Check sheet for the drawn part. Datum: minimum x, y, z corner. Units: mm. A direction names the side the tool comes from. Coordinates: 2 decimals unless noted, no trailing zeros. Order: outer loops, then holes, each group sorted by start corner. A loop starts at its lowest first (then second) coordinate and runs counter-clockwise, first axis right, second up. Notation, with made-up numbers: (87, 27.25) -> (96, 27.25) arc R15 cw to (96, 38.25) -> close; hole circle Ø3 at (-31, -21). An arc over 180 degrees is marked (long way). Answer as CSV lines item,"result".
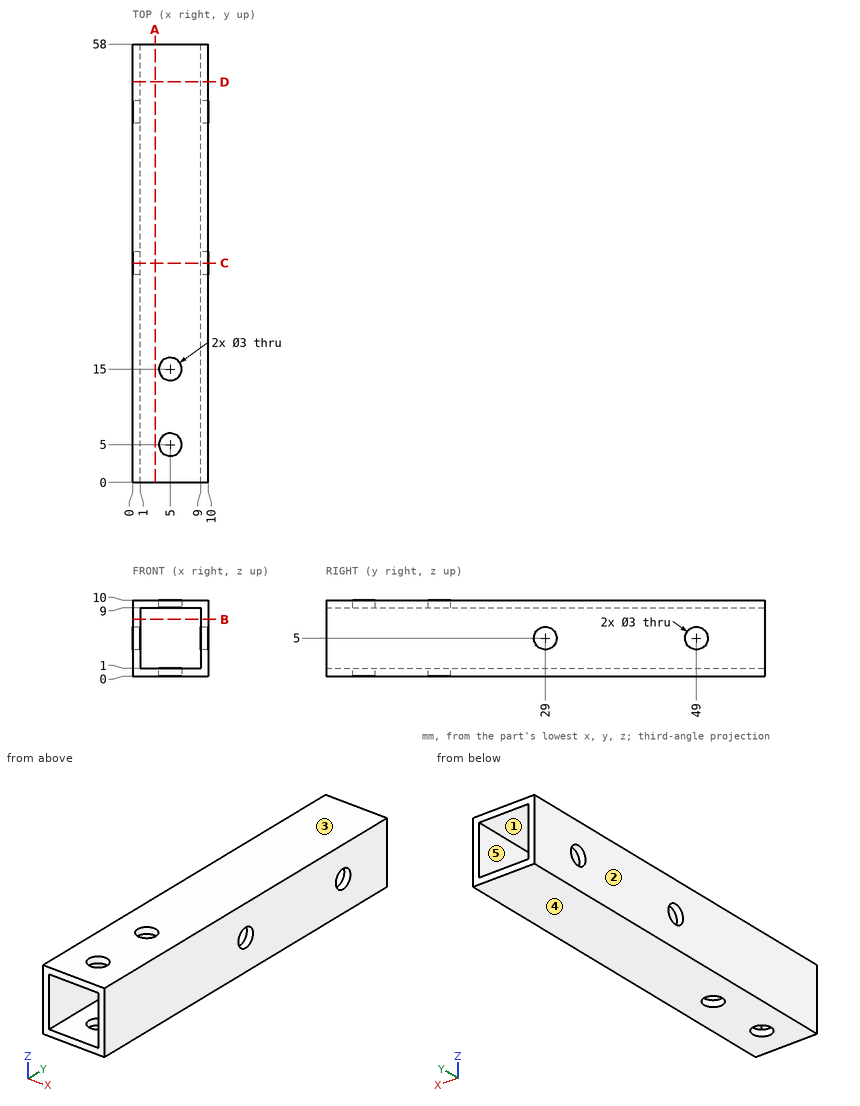
Item 1: Section check B-B, the plane z = 7.5. Record the boundary of the cut face in (x, y), plus the area to 3 significant figures.
Answer list:
outline,"(0, 0) -> (1, 0) -> (1, 58) -> (0, 58) -> close; (9, 0) -> (10, 0) -> (10, 58) -> (9, 58) -> close"
area,"116 mm2"
Item 2: Release check for a two-part mould opening along Z. For the marked faces 3, 4 and 5 record: +Z half, -Z half, draft (parallel to the pull), parting line (faces both ways), or undercut.
Answer list:
face 3,"+Z half"
face 4,"-Z half"
face 5,"undercut"
Item 3: Thickness scan on line 1 (Y direction, x = 9.7, z = 5); line 2 (Z direction, x = 4, y = 46.5). Record the ranges inside material, lowest first.
Answer list:
line 1,"0 to 27.5, 30.5 to 47.5, 50.5 to 58"
line 2,"0 to 1, 9 to 10"
Item 4: Section check D-D, the plane y = 53. Record the boundary of the cut face in (x, z), plus the area to 3 significant figures.
Answer list:
outline,"(0, 0) -> (10, 0) -> (10, 10) -> (0, 10) -> close; hole (1, 1) -> (9, 1) -> (9, 9) -> (1, 9) -> close"
area,"36.0 mm2"
Item 5: Section check A-A, the plane x = 3. Record the boundary of the cut face in (y, z).
Answer list:
outline,"(0, 0) -> (58, 0) -> (58, 1) -> (0, 1) -> close; (0, 9) -> (58, 9) -> (58, 10) -> (0, 10) -> close"
Item 6: Tool access check on the marked faces 1 and 2. Record the directions out of +Z, -Z, +X, -X, +Y, -Y that give a thin tool (end or side, any length) a straight path to the whole face; none if there is none.
Answer list:
face 1,"+Y, -Y"
face 2,"+Z, -Z, -X, +Y, -Y"
Item 7: Section check C-C, the plane y = 29. Record the boundary of the cut face in (x, z), plus the area to 3 significant figures.
Answer list:
outline,"(0, 0) -> (10, 0) -> (10, 3.5) -> (9, 3.5) -> (9, 1) -> (1, 1) -> (1, 3.5) -> (0, 3.5) -> close; (0, 6.5) -> (1, 6.5) -> (1, 9) -> (9, 9) -> (9, 6.5) -> (10, 6.5) -> (10, 10) -> (0, 10) -> close"
area,"30.0 mm2"
Item 8: Depth check by flat-ended pin: pin 1 Ø6 at (x, z) = (2, 9) entering from -Y; pin 2 Ø2.5 at (y, z) = (49, 5) entering from -X. Enter the tip coordinate at first touch or a pass-through.
Answer list:
pin 1,"y = 0"
pin 2,"through"
